The model under review builds one solid part; all positions refer to its coordinate system, in mm. A direction names the side the tool comes from. Coordinates: 2 decimals unless noted, no trailing zeros. Loops run counter-clockwise (first coordinate to the right, second up) from the corner with the lowest first, then second, coordinate; pieces in that order, holes last. Notation, with made-up numbers: M 72.25,32.25 L 90.25,32.25 A27 cw 90.25,55.25 Z; hole C 89.5,-3.75 d9. An arc over 180 degrees is marked long. Write item = value, one per line. Start each with the question number.
Q1. Wall thickness on probe 1 along X at (y, z) = (13.5, 0); probe 2 along Z at (x, y) = (-6.5, 17.5): over which ranges is each line inside the solid? List them lowest first.
Q2. For faces 1 (the face through (27, 6, -27)), 2 (the face through (-14, 2, 35)), 3 (the face through (38, 4, 0.5)), 4 (the face through (-0.5, 4, -38)), list the 3-axis set-ups (+Z, -Z, +X, -X, +Y, -Y) from which the entire face can be reached by the end or side of a thin tool; tool diameter is ignored.
Q3. We need section B-B on y = 12. Give the boundary of the cut face in (x, z).
Q4. We need section A-A on z = -11. Give the boundary of the cut face in (x, y).
Q5. Clearance check with flat-ended pins moving along their axes: pin 1 Ø0.5 at (x, z) = (0, 38.5) entering from -Y; pin 2 Ø6 at (y, z) = (12.5, 30.5) entering from +X; pin 3 Ø8 at (x, y) = (-30.5, 17.5) entering from -Z. State where each tip first meets the part, or that it passes through.
Q6. Mouldability with a two-part tool opening along Z and no side actions: class faces 5 (the face through (14.17, 3.18, -34.72)), 6 (the face through (-8.67, 13.54, 39.05)), 7 (the face through (-0.2, 25.4, 35.4)), 8 (the face through (-26.529, 4.416, 27.236)) as released by +Z, released by -Z, zero draft, split by the parting line, or undercut.
Q7. We need section C-C on x = 32. Give the boundary of the cut face in (y, z).
from build123d import *

# Parameters (mm, degrees)
SKETCH1_R           = 40
SKETCH1_R_2         = 35
BOSS_EXTRUDE1_DEPTH = 25.4
SKETCH2_R           = 37.5
SKETCH2_R_2         = 35
CUT_EXTRUDE1_DEPTH  = 4.4
SKETCH3_W           = 1
SKETCH3_H           = 6
CUT_EXTRUDE2_DEPTH  = 41
CIRPATTERN1_COUNT   = 4
CIRPATTERN1_ANGLE   = 135
SKETCH4_R           = 45.877575429
CUT_EXTRUDE3_DEPTH  = 2


with BuildPart() as part:
    # Sketch1 → Boss-Extrude1 (new body)
    with BuildSketch(Plane(origin=(0, 0, 0), x_dir=(1, 0, 0), z_dir=(0, 1, 0))):
        Circle(SKETCH1_R)
        Circle(SKETCH1_R_2, mode=Mode.SUBTRACT)
    extrude(amount=BOSS_EXTRUDE1_DEPTH)

    # Sketch2 → Cut-Extrude1 (cut)
    with BuildSketch(Plane.XZ):
        Circle(SKETCH2_R)
        Circle(SKETCH2_R_2, mode=Mode.SUBTRACT)
    extrude(amount=-CUT_EXTRUDE1_DEPTH, mode=Mode.SUBTRACT)

    # Sketch3 → Cut-Extrude2 (cut, symmetric)
    with BuildSketch(Plane.XY):
        with Locations((0, 3)):
            Rectangle(SKETCH3_W, SKETCH3_H)
    cut_extrude2 = extrude(amount=CUT_EXTRUDE2_DEPTH, both=True, mode=Mode.SUBTRACT)

    # CirPattern1: Cut-Extrude2 ×4 about axis
    cirpattern1_axis = Axis((0, 0, 0), (0, 1, 0))
    for i in range(1, CIRPATTERN1_COUNT):
        add(cut_extrude2.rotate(cirpattern1_axis, i * CIRPATTERN1_ANGLE / (CIRPATTERN1_COUNT - 1)), mode=Mode.SUBTRACT)

    # Sketch4 → Cut-Extrude3 (cut)
    with BuildSketch(Plane.XZ):
        Circle(SKETCH4_R)
    extrude(amount=-CUT_EXTRUDE3_DEPTH, mode=Mode.SUBTRACT)


solid = part.part
Returned:
q1.probe_1 = -40 to -35, 35 to 40
q1.probe_2 = -39.47 to -34.39, 34.39 to 39.47
q2.face_1 = -Y
q2.face_2 = +Z, -Z, +X, -X, -Y
q2.face_3 = +X, -X, -Y
q2.face_4 = +Z, -Z, -Y
q3.outline = C 0,0 d80; hole C 0,0 d70
q4.outline = M -38.46,2 L -35.85,2 L -35.85,4.4 L -33.23,4.4 L -33.23,25.4 L -38.46,25.4 Z; M 33.23,4.4 L 35.85,4.4 L 35.85,2 L 38.46,2 L 38.46,25.4 L 33.23,25.4 Z
q5.pin_1 = 6
q5.pin_2 = 29.05
q5.pin_3 = -29.96
q6.face_5 = undercut
q6.face_6 = split by the parting line
q6.face_7 = zero draft
q6.face_8 = undercut
q7.outline = M 2,-24 L 25.4,-24 L 25.4,-14.18 L 4.4,-14.18 L 4.4,-19.55 L 2,-19.55 Z; M 2,19.55 L 4.4,19.55 L 4.4,14.18 L 25.4,14.18 L 25.4,24 L 2,24 Z
